```python
from build123d import *

# Parameters (mm, degrees)
SKETCH_1_R          = 7.5
EXTRUDE_1_DEPTH     = 16
SKETCH_3_R          = 3.5
CUT_EXTRUDE_1_DEPTH = 57.14267539


with BuildPart() as part:
    # 草图1 → 凸台-拉伸1 (new body)
    with BuildSketch(Plane.XY):
        with BuildLine():
            Line((-21, 0), (-26, -15))
            Line((-26, -15), (-40, -15))
            Line((-40, -15), (-40, -22))
            Line((-40, -22), (40, -22))
            Line((40, -22), (40, -15))
            Line((40, -15), (26, -15))
            Line((26, -15), (21, 0))
            ThreePointArc((21, 0), (0, 21), (-21, 0))
        make_face()
        Circle(SKETCH_1_R, mode=Mode.SUBTRACT)
    extrude(amount=EXTRUDE_1_DEPTH)

    # 草图3 → 切除-拉伸1 (cut, through all)
    with BuildSketch(Plane(origin=(0, -15, 0), x_dir=(1, 0, 0), z_dir=(0, 1, 0))):
        with Locations(Location((-31.5, -8, 0), (0, 0, 180))):
            Circle(SKETCH_3_R)
        with Locations(Location((31.5, -8, 0), (0, 0, 180))):
            Circle(SKETCH_3_R)
    extrude(amount=-CUT_EXTRUDE_1_DEPTH, mode=Mode.SUBTRACT)


solid = part.part
```
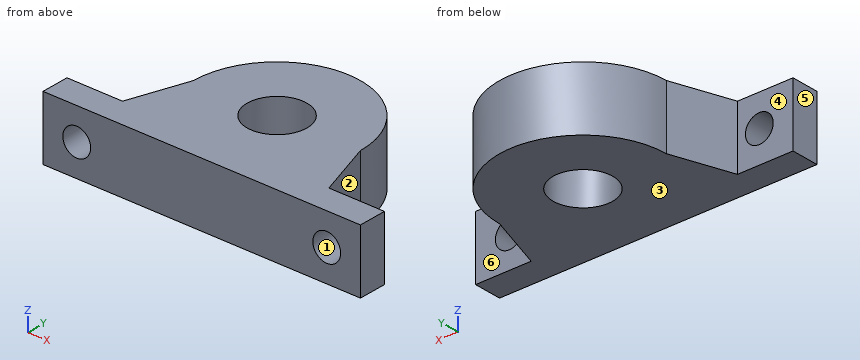
Geometry: final body of the model. Coordinates: model frame, mm. Face numbers are marked on the shaded views. A direction names the side the tool comes from. Coordinates: 2 decimals unless noted, no trailing zeros. Order: outer loops, then holes, each group sorted by start corner. A loop starts at its lowest first (then second) coordinate and runs counter-clockwise, first axis right, second up. Notation, with made-up numbers: (49.25, 31.5) - (62.25, 31.5) arc R13 cw to (62.25, 51.5) - close; hole circle Ø3 at (-34.5, -8). An arc over 180 degrees is marked (long way). Return JSON: item names as keys, results as strings. Group by question number.
1. Pull-direction query (Z, two-part tool) for the marked faces 1, 2 and 3; classes: pulls with the +Z half, pulls with the -Z half, needs draft (parallel to the pull), parting line crosses it, or undercut.
2. Set-up query: the marked faces 4, 5 and 6. Return all of +Z, -Z, +X, -X, +Y, -Y with unobstructed straight access to the full face (end or side cutting, diameter ignored); none if empty.
3. Cut plane B-B (x = 0). Output: boundary loops of the cut face in (y, z), plus the area to 3 significant figures.
4. Cut plane C-C (y = 6.5). Output: boundary loops of the cut face in (x, z).
5. Pin query (flat end, axial travel): pin 1 (1 mm diameter, centred on x = -5.5, y = 1, fed in from -Z) (3 decimals); pin 2 (7 mm diameter, centred on x = -35, z = 9.5, fed in from +Y); pin 3 (6 mm diameter, centred on x = 15, z = 11.5, fed in from +Y); pin 4 (2 mm diameter, centred on y = -4, z = 10.5, fed in from +X). Return the tip coordinate at first contact, or that it passes through.
6. Material intervals for line 1 along Y through (x, z) = (0, 3.25); line 2 along X through (y, z) = (-19.5, 10.5); line 3 along Y through (x, z) = (36.5, 10.25), sorted ascending. Write a range as [from, to].
7. Cut plane A-A (z = 8). Output: boundary loops of the cut face in (x, y).
8. Cut plane D-D (z = 14.25). Output: boundary loops of the cut face in (x, y).
Resolved:
{
 "1": {"face 1": "undercut", "face 2": "needs draft", "face 3": "pulls with the -Z half"},
 "2": {"face 4": "+Z, -Z, -X, +Y", "face 5": "+Z, -Z, -X, +Y, -Y", "face 6": "+Z, -Z, +X, +Y"},
 "3": {"outline": "(-22, 0) - (-7.5, 0) - (-7.5, 16) - (-22, 16) - close; (7.5, 0) - (21, 0) - (21, 16) - (7.5, 16) - close", "area": "448 mm²"},
 "4": {"outline": "(-19.97, 0) - (-3.74, 0) - (-3.74, 16) - (-19.97, 16) - close; (3.74, 0) - (19.97, 0) - (19.97, 16) - (3.74, 16) - close"},
 "5": {"pin 1": "passes through", "pin 2": "stops at y = -15", "pin 3": "stops at y = 17.23", "pin 4": "stops at x = 22.67"},
 "6": {"line 1": "y = [-22, -7.5], [7.5, 21]", "line 2": "x = [-40, -33.95], [-29.05, 29.05], [33.95, 40]", "line 3": "y = [-22, -15]"},
 "7": {"outline": "(-40, -22) - (-35, -22) - (-35, -15) - (-40, -15) - close; (-28, -22) - (28, -22) - (28, -15) - (26, -15) - (21, 0) arc R21 ccw to (-21, 0) - (-26, -15) - (-28, -15) - close; (35, -22) - (40, -22) - (40, -15) - (35, -15) - close; hole circle Ø15 at (0, 0)"},
 "8": {"outline": "(-40, -22) - (40, -22) - (40, -15) - (26, -15) - (21, 0) arc R21 ccw to (-21, 0) - (-26, -15) - (-40, -15) - close; hole circle Ø15 at (0, 0)"}
}
